Model file for the job. Use its own axes, mm. Face numbers are marked on the shaded views. A direction names the side the tool comes from. Give positions to 0.01 mm unless a question says otherwise; leave off trailing zeros. Write each loop counter-clockwise with the first axis right and the second up, starting at its lowest first coordinate (ties: lowest second). Pieces come first, ordered by that corner, then holes. Notation, with made-up numbers: M 30,15.5 L 70,15.5 A26 ccw 70,50.5 Z; hole C -4.5,26.25 d3. An arc over 180 degrees is marked long. Answer as a JSON object with one key per item and string values. Group by question number.
```python
from build123d import *

# Parameters (mm, degrees)
EXTRUDE_1_DEPTH          = 25
SHELL_2_T                = -3
SKETCH_3_R               = 2.5
EXTRUDE_4_DEPTH          = 20
CUT_EXTRUDE_4_DEPTH      = 212.557459677
CUT_EXTRUDE_4_DEPTH_BACK = 212.557459677
SKETCH_4_R               = 1.5


with BuildPart() as part:
    # 草图1 → 凸台-拉伸1 (new body)
    with BuildSketch(Plane.XY):
        with BuildLine():
            Line((-193.42519685, 70), (-168.42519685, 70))
            ThreePointArc((-168.42519685, 70), (-164.889662944, 68.535533906), (-163.42519685, 65))
            Line((-163.42519685, 65), (-163.42519685, 5))
            ThreePointArc((-163.42519685, 5), (-164.889662944, 1.464466094), (-168.42519685, 0))
            Line((-168.42519685, 0), (-193.42519685, 0))
            ThreePointArc((-193.42519685, 0), (-196.960730756, 1.464466094), (-198.42519685, 5))
            Line((-198.42519685, 5), (-198.42519685, 65))
            ThreePointArc((-198.42519685, 65), (-196.960730756, 68.535533906), (-193.42519685, 70))
        make_face()
    extrude(amount=EXTRUDE_1_DEPTH)

    # 抽壳2
    shell_2_openings = [part.faces().sort_by_distance(p)[0] for p in [
        (-180.92519685, 35, 25),
    ]]
    offset(amount=SHELL_2_T, openings=shell_2_openings, kind=Kind.INTERSECTION)

    # 草图3 → 凸台-拉伸4 (add)
    with BuildSketch(Plane.XY.offset(3)):
        with Locations((-192.656739456, 62.5)):
            Circle(SKETCH_3_R)
        with Locations((-192.656739456, 7.5)):
            Circle(SKETCH_3_R)
        with Locations((-169.193654245, 62.5)):
            Circle(SKETCH_3_R)
        with Locations((-169.193654245, 7.5)):
            Circle(SKETCH_3_R)
    extrude(amount=EXTRUDE_4_DEPTH)

    # 草图4 → 切除-拉伸4 (cut, two sides: drawn at the far end of the back side and taken through both)
    with BuildSketch(Plane.XY.offset(3).offset(-CUT_EXTRUDE_4_DEPTH_BACK)):
        with Locations((-192.656739456, 62.5)):
            Circle(SKETCH_4_R)
        with Locations((-169.193654245, 62.5)):
            Circle(SKETCH_4_R)
        with Locations((-169.193654245, 7.5)):
            Circle(SKETCH_4_R)
        with Locations((-192.656739456, 7.5)):
            Circle(SKETCH_4_R)
    extrude(amount=CUT_EXTRUDE_4_DEPTH + CUT_EXTRUDE_4_DEPTH_BACK, mode=Mode.SUBTRACT)


solid = part.part
```
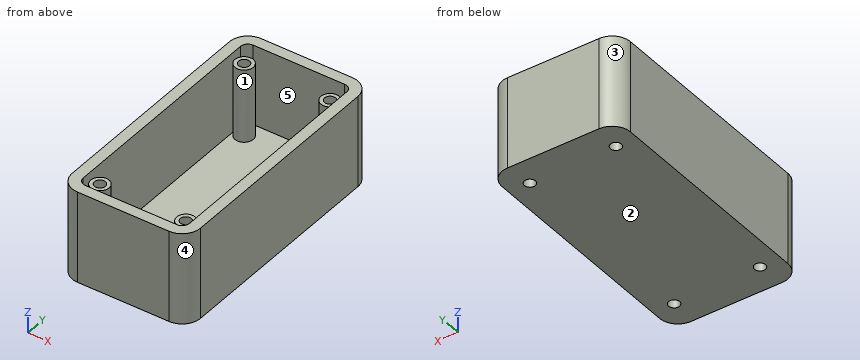
Q1. Drop flat-ended pins along their axis: P1, Ø1.8, axis at x = -169.19, y = 7.5, coming from the +Z side; P2, Ø5.5, axis at x = -170, y = 7, coming from the +Z side; P3, Ø1, axis at x = -170.5, y = 46, coming from the +Z side; P4, Ø4, axis at x = -194, y = 19.5, coming from the +Z side. Give the stop position or say it passes through.
Q2. Two-plate mould, pull along X, no slides. Class the marked faces 3, 4 and 5: +X half, -X half, draft (parallel to the pull), parting line (faces both ways), or undercut.
Q3. 3-axis set-ups, long thin cutter, end or side, ignore diameter. For the marked faces 1 and 2: which of +Z, -Z, +X, -X, +Y, -Y reach the whole face in a straight line?
Q4. Slice it at A-A, the plane z = 15. Count the separate pieces of the cut face and the enclosed holes in it, then the cut area to 3 significant figures.
Q5. Wall check: L1, parallel to Y at x = -183.5, z = 23.5; L2, parallel to Y at x = -169, z = 19.5; L3, parallel to X at y = 54.5, z = 19.75. Give the ranges that are in metal, low to high.
Q6. Slice it at B-B, the plane y = 62.5. Write the cut outline in (x, z), then the cut area to 3 significant figures.
Q7. Slice it at D-D, the plane x = -192. Write the cut outline in (y, z).
Q8. Slice it at C-C, the plane x = -188.5. Write the cut outline in (y, z).
Solved:
{
 "1": {"P1": "passes through", "P2": "stops at z = 23", "P3": "stops at z = 3", "P4": "stops at z = 25"},
 "2": {"face 3": "-X half", "face 4": "+X half", "face 5": "undercut"},
 "3": {"face 1": "+Z", "face 2": "-Z, +X, -X, +Y, -Y"},
 "4": {"separate pieces": "5", "enclosed holes": "5", "area": "626 mm²"},
 "5": {"L1": "y = 0 to 3, 67 to 70", "L2": "y = 0 to 3, 5.01 to 6.01, 8.99 to 9.99, 60.01 to 61.01, 63.99 to 64.99, 67 to 70", "L3": "x = -198.43 to -195.43, -166.43 to -163.43"},
 "6": {"outline": "M -198.43,0 L -194.16,0 L -194.16,23 L -195.16,23 L -195.16,3 L -195.43,3 L -195.43,25 L -198.43,25 Z; M -191.16,0 L -170.69,0 L -170.69,23 L -171.69,23 L -171.69,3 L -190.16,3 L -190.16,23 L -191.16,23 Z; M -167.69,0 L -163.43,0 L -163.43,25 L -166.43,25 L -166.43,3 L -166.69,3 L -166.69,23 L -167.69,23 Z", "area": "299 mm²"},
 "7": {"outline": "M 0,0 L 6.15,0 L 6.15,23 L 5.09,23 L 5.09,3 L 3,3 L 3,25 L 0,25 Z; M 8.85,0 L 61.15,0 L 61.15,23 L 60.09,23 L 60.09,3 L 9.91,3 L 9.91,23 L 8.85,23 Z; M 63.85,0 L 70,0 L 70,25 L 67,25 L 67,3 L 64.91,3 L 64.91,23 L 63.85,23 Z"},
 "8": {"outline": "M 0,0 L 70,0 L 70,25 L 67,25 L 67,3 L 3,3 L 3,25 L 0,25 Z"}
}
